Work out the finished part from the listing and answer in its coordinate system (mm). A direction names the side the tool comes from. Coordinates: 2 decimals unless noted, no trailing zeros. Loops run counter-clockwise (first coordinate to the right, second up) from the corner with the lowest first, then second, coordinate; pieces in that order, holes last. Notation, with made-up numbers: (41.25, 6.25) -> (61.25, 6.25) arc R11 cw to (61.25, 26.25) -> close; hole circle Ø5 at (59.5, -10.75). An arc over 180 degrees is marked (long way). Answer as CSV lines item,"result".
```python
from build123d import *

# Parameters (mm, degrees)
SKETCH1_R           = 0.75
BOSS_EXTRUDE1_DEPTH = 3.5
CIRPATTERN1_COUNT   = 4
SKETCH3_W           = 4
SKETCH3_H           = 4
SKETCH3_W_2         = 1.5
SKETCH3_H_2         = 1.5
BOSS_EXTRUDE2_DEPTH = 2
FILLET1_R           = 0.5


with BuildPart() as part:
    # Sketch1 → Boss-Extrude1 (new, symmetric)
    with BuildSketch(Plane.XY):
        Circle(SKETCH1_R)
    boss_extrude1 = extrude(amount=BOSS_EXTRUDE1_DEPTH, both=True)

    # CirPattern1: Boss-Extrude1 ×4 about axis
    cirpattern1_axis = Axis((0, -1.485, 0), (0, 1, 0))
    for i in range(1, CIRPATTERN1_COUNT):
        add(boss_extrude1.rotate(cirpattern1_axis, i * 360 / CIRPATTERN1_COUNT))

    # Sketch3 → Boss-Extrude2 (add, symmetric)
    with BuildSketch(Plane(origin=(0, 0, 0), x_dir=(1, 0, 0), z_dir=(0, 1, 0))):
        Rectangle(SKETCH3_W, SKETCH3_H)
        Rectangle(SKETCH3_W_2, SKETCH3_H_2, mode=Mode.SUBTRACT)
        Rectangle(SKETCH3_W_2, SKETCH3_H_2)
    extrude(amount=BOSS_EXTRUDE2_DEPTH, both=True)

    # Fillet1
    fillet1_edges = [part.edges().sort_by_distance(p)[0] for p in [
        (0, 2, 2),
        (-2, 0, 2),
        (2, -2, 0),
        (2, 0, 2),
        (0, -2, -2),
        (2, 0, -2),
        (-2, 2, 0),
        (-2, 0, -2),
        (2, 2, 0),
        (0, 2, -2),
        (0, -2, 2),
        (-2, -2, 0),
    ]]
    fillet(fillet1_edges, radius=FILLET1_R)


solid = part.part
```
(1) A cutting plane is placed at C-C, the plane x = 0. Write down the section's boundary in (y, z).
Computed values:
outline,"(-2, -1.5) arc R0.5 ccw to (-1.5, -2) -> (-0.75, -2) -> (-0.75, -3.5) -> (0.75, -3.5) -> (0.75, -2) -> (1.5, -2) arc R0.5 ccw to (2, -1.5) -> (2, 1.5) arc R0.5 ccw to (1.5, 2) -> (0.75, 2) -> (0.75, 3.5) -> (-0.75, 3.5) -> (-0.75, 2) -> (-1.5, 2) arc R0.5 ccw to (-2, 1.5) -> close"
(2) Which of the six approach directions +Z, -Z, +X, -X, +Y, -Y give full straight-line access (tool end or side, diameter ignored) to faces 1 (the face through (-0.75, 0.03, 2.76)), 2 (the face through (2, 0, 1)), 3 (the face through (3.5, 0, 0)), 4 (the face through (-1, 0, -2)), 5 (the face through (-2, 0, 1))?
Computed values:
face 1,"+Z"
face 2,"+X"
face 3,"+Z, -Z, +X, +Y, -Y"
face 4,"-Z"
face 5,"-X"
(3) A cutting plane is placed at D-D, the plane z = 0. Write down the section's boundary in (x, y), and give its area (3 significant figures).
Computed values:
outline,"(-3.5, -0.75) -> (-2, -0.75) -> (-2, -1.5) arc R0.5 ccw to (-1.5, -2) -> (1.5, -2) arc R0.5 ccw to (2, -1.5) -> (2, -0.75) -> (3.5, -0.75) -> (3.5, 0.75) -> (2, 0.75) -> (2, 1.5) arc R0.5 ccw to (1.5, 2) -> (-1.5, 2) arc R0.5 ccw to (-2, 1.5) -> (-2, 0.75) -> (-3.5, 0.75) -> close"
area,"20.3 mm2"
(4) Consider line 1 along X through (y, z) = (0.8, 0.25); line 2 along X through (y, z) = (-0.8, 1.75). Determine where each line is inside the solid, lowest interval first.
Computed values:
line 1,"-2 to 2"
line 2,"-1.93 to 1.93"
(5) A cutting plane is placed at A-A, the plane z = 1.25. Write down the section's boundary in (x, y).
Computed values:
outline,"(-2, -1.5) arc R0.5 ccw to (-1.5, -2) -> (1.5, -2) arc R0.5 ccw to (2, -1.5) -> (2, 1.5) arc R0.5 ccw to (1.5, 2) -> (-1.5, 2) arc R0.5 ccw to (-2, 1.5) -> close"
